from build123d import *

# Parameters (mm, degrees)
SKETCH_1_R      = 9
SKETCH_1_R_2    = 1.5
EXTRUDE_1_DEPTH = 5
FILLET_1_R      = 2
CHAMFER_1_SIZE  = 10
FILLET_3_R      = 10


with BuildPart() as part:
    # 草图1 → 凸台-拉伸1 (new body)
    with BuildSketch(Plane(origin=(0, 0, 0), x_dir=(1, 0, 0), z_dir=(0, 1, 0))):
        with BuildLine():
            Line((5, 17.339745962), (5, 65))
            ThreePointArc((5, 65), (0, 70), (-5, 65))
            Line((-5, 65), (-5, 17.339745962))
            Line((-5, 17.339745962), (-22.516660498, -13))
            Line((-22.516660498, -13), (22.516660498, -13))
            Line((22.516660498, -13), (5, 17.339745962))
        make_face()
        with Locations(Location((0, 0, 0), (0, 0, 270))):
            Circle(SKETCH_1_R, mode=Mode.SUBTRACT)
        with Locations(Location((0, 20, 0), (0, 0, 270))):
            Circle(SKETCH_1_R_2, mode=Mode.SUBTRACT)
        with Locations(Location((-17.320508076, -10, 0), (0, 0, 270))):
            Circle(SKETCH_1_R_2, mode=Mode.SUBTRACT)
        with Locations(Location((17.320508076, -10, 0), (0, 0, 270))):
            Circle(SKETCH_1_R_2, mode=Mode.SUBTRACT)
    extrude(amount=EXTRUDE_1_DEPTH)

    # 圆角1
    fillet_1_edges = [part.edges().sort_by_distance(p)[0] for p in [
        (22.516660498, 2.5, 13),
        (-22.516660498, 2.5, 13),
    ]]
    fillet(fillet_1_edges, radius=FILLET_1_R)

    # 倒角1
    chamfer_1_edges = [part.edges().sort_by_distance(p)[0] for p in [
        (-5, 2.5, -17.339745962),
        (5, 2.5, -17.339745962),
    ]]
    chamfer(chamfer_1_edges, length=CHAMFER_1_SIZE)

    # 圆角3
    fillet_3_edges = [part.edges().sort_by_distance(p)[0] for p in [
        (5, 2.5, -27.339745962),
        (10, 2.5, -8.679491924),
        (-10, 2.5, -8.679491924),
        (-5, 2.5, -27.339745962),
    ]]
    fillet(fillet_3_edges, radius=FILLET_3_R)


solid = part.part
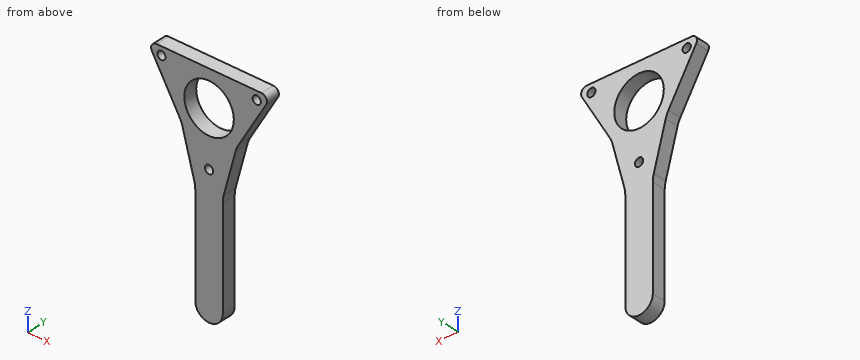
Build history of the part. All positions in model axes, mm. Coordinates: 2 decimals unless noted, no trailing zeros. Write each loop counter-clockwise with the first axis right and the second up, starting at its lowest first coordinate (ties: lowest second). Pieces come first, ordered by that corner, then holes. Notation, with made-up numbers: (58, 20) -> (101, 20) arc R16 ccw to (101, 49) -> close; hole circle Ø6 at (50, 51.5). An arc over 180 degrees is marked (long way). Use CSV: the item, a comma, the result in double quotes. Start each with the question number.
Q1. Flat gauge pins, fed straight in: pin 1 Ø3 at (y, z) = (2, -41.5) entering from +X; pin 2 Ø2.5 at (x, z) = (17.32, 10) entering from +Y; pin 3 Ø8 at (x, z) = (-12, -16) entering from -Y. Where does each tip first touch, or does it go through?
Q2. Cut at D-D, the plane y = 2. List the corners of the cut face in (x, z), then the cut area to 3 significant figures.
Q3. Drill centre lines: probe 1 along Z at (x, y) = (1, 4.55); probe 2 along X at (y, z) = (3.35, -19); probe 3 along X at (y, z) = (4.65, -38.5). Where is each one in solid material? Low to high.
Q4. Cut at C-C, the plane x = 7.5. List the corners of the cut face in (y, z).
Q5. Cut at A-A, the plane x = 0. List the corners of the cut face in (y, z), then the cut area to 3 significant figures.
Q6. Cut at B-B, the plane z = -20. List the corners of the cut face in (x, y).
Checked values:
1,pin 1,"stops at x = 5"
1,pin 2,"passes through"
1,pin 3,"stops at y = 0"
2,outline,"(-20.78, 10) -> (-10.66, -7.54) arc R10 cw to (-9.66, -9.95) -> (-5.34, -26.07) arc R10 cw to (-5, -28.66) -> (-5, -65) arc R5 ccw to (5, -65) -> (5, -28.66) arc R10 cw to (5.34, -26.07) -> (9.66, -9.95) arc R10 cw to (10.66, -7.54) -> (20.78, 10) arc R2 ccw to (19.05, 13) -> (-19.05, 13) arc R2 ccw to start; hole circle Ø3 at (-17.32, 10); hole circle Ø18 at (0, 0); hole circle Ø3 at (0, -20); hole circle Ø3 at (17.32, 10)"
2,area,"1,120 mm²"
3,probe 1,"z = -69.9 to -21.12, -18.88 to -8.94, 8.94 to 13"
3,probe 2,"x = -7.23 to -1.12, 1.12 to 7.23"
3,probe 3,"x = -5 to 5"
4,outline,"(0, -18.01) -> (5, -18.01) -> (5, -4.97) -> (0, -4.97) -> close; (0, 4.97) -> (5, 4.97) -> (5, 13) -> (0, 13) -> close"
5,outline,"(0, -70) -> (5, -70) -> (5, -21.5) -> (0, -21.5) -> close; (0, -18.5) -> (5, -18.5) -> (5, -9) -> (0, -9) -> close; (0, 9) -> (5, 9) -> (5, 13) -> (0, 13) -> close"
5,area,"310 mm²"
6,outline,"(-6.97, 0) -> (-1.5, 0) -> (-1.5, 5) -> (-6.97, 5) -> close; (1.5, 0) -> (6.97, 0) -> (6.97, 5) -> (1.5, 5) -> close"
